Source: CAD feature listing. Evaluate the final solid. Frame: model axes, mm. A direction names the side the tool comes from. Round coordinates to 2 decimals unless told otherwise and drop trailing zeros. Order: outer loops, then holes, each group sorted by start corner. A loop starts at its lowest first (then second) coordinate and runs counter-clockwise, first axis right, second up. Notation, with made-up numbers: M 63.25,39.25 L 113.25,39.25 A9 ccw 113.25,53.25 Z; hole C 56.5,56.5 d1. An arc over 180 degrees is marked long. Answer in a Markdown table with one row per item. Add a question column.
```python
from build123d import *

# Parameters (mm, degrees)
BOSS_EXTRUDE1_DEPTH   = 40
CHAMFER1_SIZE         = 1.5
CHAMFER2_SIZE         = 3
F_6_32_TAPPED_HOLE1_D = 2.7051
F_6_CLEARANCE_HOLE1_D = 3.6576


with BuildPart() as part:
    # Sketch1 → Boss-Extrude1 (new body, symmetric)
    with BuildSketch(Plane(origin=(0, 0, 0), x_dir=(0, 0, -1), z_dir=(1, 0, 0))):
        Polygon((0, 0), (31.75, 0), (31.75, 3.175), (3.175, 3.175), (3.175, 31.75), (0, 31.75), align=None)
    extrude(amount=BOSS_EXTRUDE1_DEPTH, both=True)

    # Chamfer1
    chamfer1_edges = [part.edges().sort_by_distance(p)[0] for p in [
        (0, 31.75, -3.175),
        (0, 3.175, -3.175),
        (0, 3.175, -31.75),
    ]]
    chamfer(chamfer1_edges, length=CHAMFER1_SIZE)

    # Chamfer2
    chamfer2_edges = [part.edges().sort_by_distance(p)[0] for p in [
        (-40, 31.75, -0.8375),
        (-40, 0.8375, -31.75),
        (40, 0.8375, -31.75),
        (40, 31.75, -0.8375),
    ]]
    chamfer(chamfer2_edges, length=CHAMFER2_SIZE)

    # #6-32 Tapped Hole1 (through all)
    with Locations(Plane(origin=(0, 3.175, 0), x_dir=(1, 0, 0), z_dir=(0, 1, 0))):
        with Locations((-37.208, 27.221), (10.792, 27.221), (-5.208, 27.221), (-13.208, 19.221), (-21.208, 27.221), (18.792, 19.221), (26.792, 27.221)):
            Hole(F_6_32_TAPPED_HOLE1_D / 2)

    # #6 Clearance Hole1 (through all)
    with Locations(Plane(origin=(0, 0, -3.175), x_dir=(-1, 0, 0), z_dir=(0, 0, -1))):
        with Locations((-10.792, 16), (-18.792, 8), (-18.792, 24), (-26.792, 16), (13.208, 24), (5.208, 16), (13.208, 8), (21.208, 16)):
            Hole(F_6_CLEARANCE_HOLE1_D / 2)


solid = part.part
```
(1) Access query for faces 1 (the face through (-5.604, 14.215, -1.565)), 2 (the face through (1, 3.175, -18)). Directions: +Z, -Z, +X, -X, +Y, -Y. A direction counts if a zero-diameter tool reaches every point of the face in a straight line with its end or side. Return the directions, or none.
(2) Cut plane C-C (x = -10). Return loops of the section in (y, z) (3 decimals).
(3) Cut plane D-D (z = -21.5). Return loops of the section in (x, y) (3 decimals), and give its area (3 significant figures).
(4) Pin query (flat end, axial travel): pin 1 (4.5 mm diameter, centred on x = 10.792, z = -27.221, fed in from +Y) (3 decimals); pin 2 (7.5 mm diameter, centred on x = -12.5, y = 15, fed in from -Z) (3 decimals). Return the tip coordinate at first contact, or that it passes through.
(5) Line query: line 1 (Y direction, x = -13, z = -27) (3 decimals); line 2 (Z direction, x = -5, y = 11) (3 decimals); line 3 (Z direction, x = -7, y = 4). Output: solid intervals per line, ascending. Write a range as from..to.
(6) Cut plane B-B (y = 16). Return loops of the section in (x, z) (3 decimals), and give its area (3 significant figures).
(7) Draft query along X for faces 3 (the face through (10.17, 1.57, -26.02)), 4 (the face through (40, 8, -3)), 5 (the face through (-38.52, 30.23, -1.61)). Return one class per face: +X half, -X half, draft (parallel to the pull), parting line (faces both ways), or undercut.
(8) Cut plane A-A (y = 24). Return loops of the section in (x, z) (3 decimals).
Answer list:
| question | item | result |
|---|---|---|
| 1 | face 1 | +Z, -Z |
| 1 | face 2 | -Z, +X, -X, +Y |
| 2 | outline | M 0,-31.75 L 1.675,-31.75 L 3.175,-30.25 L 3.175,-4.675 L 4.675,-3.175 L 30.25,-3.175 L 31.75,-1.675 L 31.75,0 L 0,0 Z |
| 3 | outline | M -40,0 L 40,0 L 40,3.175 L -40,3.175 Z |
| 3 | area | 254 mm² |
| 4 | pin 1 | y = 3.175 |
| 4 | pin 2 | z = -3.175 |
| 5 | line 1 | 0..3.175 |
| 5 | line 2 | -3.175..0 |
| 5 | line 3 | -3.85..0 |
| 6 | outline | M -40,-3.175 L -23.037,-3.175 L -23.037,0 L -40,0 Z; M -19.379,-3.175 L -7.037,-3.175 L -7.037,0 L -19.379,0 Z; M -3.379,-3.175 L 8.963,-3.175 L 8.963,0 L -3.379,0 Z; M 12.621,-3.175 L 24.963,-3.175 L 24.963,0 L 12.621,0 Z; M 28.621,-3.175 L 40,-3.175 L 40,0 L 28.621,0 Z |
| 6 | area | 208 mm² |
| 7 | face 3 | undercut |
| 7 | face 4 | +X half |
| 7 | face 5 | -X half |
| 8 | outline | M -40,-3.175 L -15.037,-3.175 L -15.037,0 L -40,0 Z; M -11.379,-3.175 L 16.963,-3.175 L 16.963,0 L -11.379,0 Z; M 20.621,-3.175 L 40,-3.175 L 40,0 L 20.621,0 Z |
